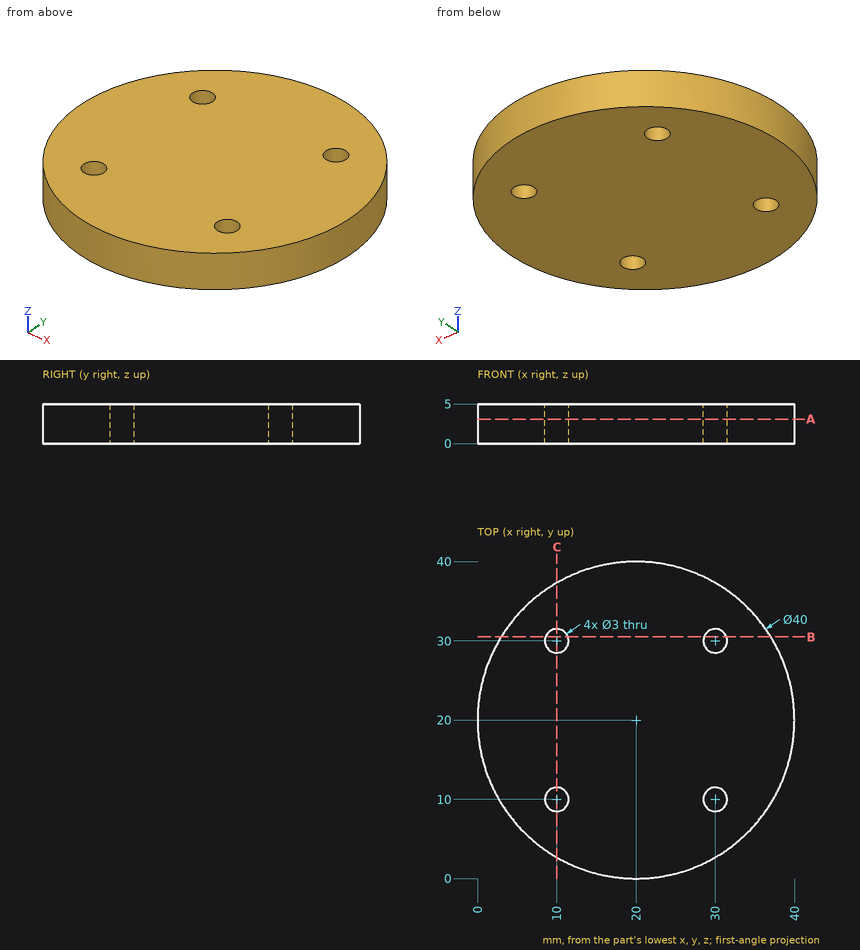
Verification items for this drawing (mm, ordinates from the low corner). Coordinates: 2 decimals unless noted, no trailing zeros. Write each loop counter-clockwise with the first axis right and the second up, starting at its lowest first coordinate (ties: lowest second). Pieces come first, ordered by that corner, then holes. Notation, with made-up numbers: M -25,78 L -7,78 A19 cw -7,106 Z; hole C 39.25,79.5 d9. An arc over 180 degrees is marked long. Answer as CSV lines item,"result".
Q1. Cross-section at C-C (x = 10). Record the boundary of the cut face in (y, z), then the cut area to 3 significant figures.
Check result:
outline,"M 2.68,0 L 8.5,0 L 8.5,5 L 2.68,5 Z; M 11.5,0 L 28.5,0 L 28.5,5 L 11.5,5 Z; M 31.5,0 L 37.32,0 L 37.32,5 L 31.5,5 Z"
area,"143 mm^2"
Q2. Go/stop test with flat-tipped pins: pin 1 (5 mm diameter, centred on x = 30, y = 30, fed in from -Z); pin 2 (2.5 mm diameter, centred on x = 30, y = 10, fed in from -Z); pin 3 (1.5 mm diameter, centred on y = 28.5, z = 1.5, fed in from -X); pin 4 (3 mm diameter, centred on x = 15, z = 1, fed in from +Y). Record where each tip stops, or that it passes through.
Check result:
pin 1,"z = 0"
pin 2,"through"
pin 3,"x = 1.56"
pin 4,"y = 39.69"
Q3. Material ranges on probe 1 along Y at (x, z) = (10, 3.25); probe 2 along X at (y, z) = (10.5, 1.55); probe 3 along X at (y, z) = (16, 2.25), recorded low to high. Write a range as from..to.
Check result:
probe 1,"2.68..8.5, 11.5..28.5, 31.5..37.32"
probe 2,"2.4..8.59, 11.41..28.59, 31.41..37.6"
probe 3,"0.4..39.6"
Q4. Cross-section at A-A (z = 3.1). Record the boundary of the cut face in (x, y).
Check result:
outline,"C 20,20 d40; hole C 10,10 d3; hole C 10,30 d3; hole C 30,10 d3; hole C 30,30 d3"
Q5. Cross-section at B-B (y = 30.5). Record the boundary of the cut face in (x, z), then the cut area to 3 significant figures.
Check result:
outline,"M 2.98,0 L 8.59,0 L 8.59,5 L 2.98,5 Z; M 11.41,0 L 28.59,0 L 28.59,5 L 11.41,5 Z; M 31.41,0 L 37.02,0 L 37.02,5 L 31.41,5 Z"
area,"142 mm^2"
